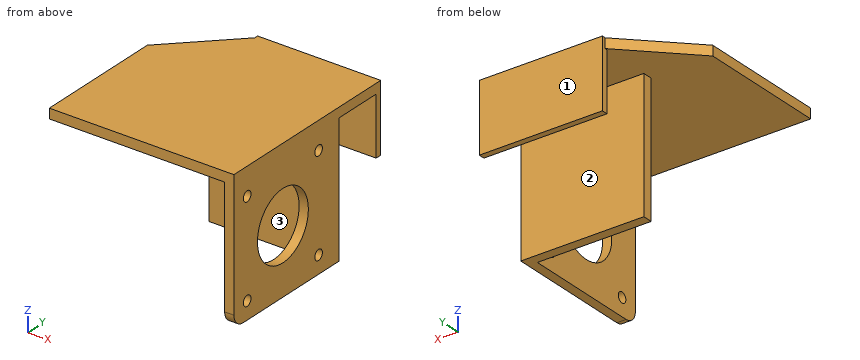
Solid Edge part; units mm, degrees
sketch "Sketch1" plane through (0, 0, 0) normal (1, 0, 0) x (0, 1, 0)
  circle A0 centre (-15.5, -15.5) radius 1.65
  circle A1 centre (0, 0) radius 11.05
  circle A2 centre (15.5, 15.5) radius 1.65
  line L0 (-21.25, 21.25) -> (21.25, 21.25)
  line L1 (21.25, 21.25) -> (21.25, -21.25)
  line L2 (21.25, -21.25) -> (-21.25, -21.25)
  line L3 (-21.25, -21.25) -> (-21.25, 21.25)
  circle A3 centre (-15.5, 15.5) radius 1.65
  circle A4 centre (15.5, -15.5) radius 1.65
extrude "Protrusion1" add sketch "Sketch1" against normal blind 3
sketch "Sketch2" plane through (0, 0, 0) normal (1, 0, 0) x (0, 1, 0)
  line L0 (24.45, -21.25) -> (21.25, -21.25)
  line L1 (21.25, 21.25) -> (21.25, -21.25)
  line L2 (21.25, 21.25) -> (21.25, 24.45)
  line L3 (-21.25, 24.45) -> (42.45, 24.45)
  line L4 (42.45, 24.45) -> (42.45, 2.25)
  line L5 (42.45, 2.25) -> (40.45, 2.25)
  line L6 (40.45, 2.25) -> (40.45, 21.25)
  line L7 (40.45, 21.25) -> (24.45, 21.25)
  line L8 (24.45, 21.25) -> (24.45, -21.25)
extrude "Fensterklammer" add sketch "Sketch2" against normal blind 40 material side at (0, 22.85, -21.2)
sketch "Sketch3" plane through (0, 0, 0) normal (1, 0, 0) x (0, 1, 0)
  line L0 (-21.25, 24.45) -> (42.45, 24.45)
  line L1 (21.25, 21.25) -> (21.25, 24.45)
  line L2 (-21.25, 21.25) -> (21.25, 21.25)
  line L3 (-21.25, 21.25) -> (-21.25, 24.45)
extrude "Elektonik_Halter" add sketch "Sketch3" against normal blind 60 material side at (0, 10.6, 24.4)
sketch "Sketch4" plane through (-31.5, 0, 21.25) normal (0, 0, -1) x (0, -1, 0)
  line L0 (-41.25, 8.5) -> (-21.25, 8.5)
  line L1 (-21.25, 8.5) -> (-21.25, 28.5)
  line L2 (-41.25, 8.5) -> (-21.25, 28.5)
extrude "Protrusion2" add sketch "Sketch4" against normal up to vertex (3.2 mm away)
fillet "R4" radius 4 1 edges at (-1.5, -21.25, -21.25)
Read the model definition and answer for the solid it produces. Units are mm, in the model's axes. Face numbers are marked on the shaded views. A direction names the side the tool comes from. Round coordinates to 2 decimals unless told otherwise and drop trailing zeros. Write each loop counter-clockwise with the first axis right and the second up, starting at its lowest first coordinate (ties: lowest second). Pieces come first, ordered by that corner, then holes.
1. The part is cut by section C-C, the plane z = -15.5. Determine the outline of the cut face in (x, y).
2. The part is cut by section D-D, the plane y = 0. Determine the outline of the cut face in (x, z).
3. Given pin 1 Ø3 at (y, z) = (-15.5, -15.5) entering from -X; pin 2 Ø6 at (y, z) = (-3, 18.5) entering from +X; pin 3 Ø1 at (x, y) = (-21.5, 41.5) entering from -Z; pin 4 Ø1.6 at (y, z) = (41.5, 17.5) entering from -X, each flat-ended and moving along its own axis, determine where each tip first touches the part or whether it passes through.
4. The part is cut by section A-A, the plane z = 19. Determine the outline of the cut face in (x, y), then the cut area to 4 significant figures.
5. Straight lines are drawn through the part: L1, parallel to Z at x = -1, y = 15.5; L2, parallel to Y at x = -2, z = -15; L3, parallel to Y at x = -39, z = 19.5. For each, find the intervals that lie inside material, in ascending order.
6. The part is cut by section B-B, the plane y = 15.5. Determine the outline of the cut face in (x, z), then the cut area to 3 significant figures.
7. Which of the six approach directions +Z, -Z, +X, -X, +Y, -Y give full straight-line access (tool end or side, diameter ignored) to the marked faces 1, 2 and 3?
Values:
1. outline: (-40, 21.25) - (-3, 21.25) - (-3, 17.15) - (0, 17.15) - (0, 24.45) - (-40, 24.45) - close; (-3, -21.25) - (0, -21.25) - (0, -17.15) - (-3, -17.15) - close; (-3, -13.85) - (0, -13.85) - (0, 13.85) - (-3, 13.85) - close
2. outline: (-60, 21.25) - (-3, 21.25) - (-3, 11.05) - (0, 11.05) - (0, 24.45) - (-60, 24.45) - close; (-3, -21.25) - (0, -21.25) - (0, -11.05) - (-3, -11.05) - close
3. pin 1: passes through
3. pin 2: stops at x = 0
3. pin 3: stops at z = 2.25
3. pin 4: stops at x = -40
4. outline: (-40, 21.25) - (-3, 21.25) - (-3, -21.25) - (0, -21.25) - (0, 24.45) - (-40, 24.45) - close; (-40, 40.45) - (0, 40.45) - (0, 42.45) - (-40, 42.45) - close
4. area: 335.5 mm2
5. L1: z = -21.25 to -17.15, -13.85 to 13.85, 17.15 to 24.45
5. L2: y = -21.25 to -17.07, -13.93 to 13.93, 17.07 to 24.45
5. L3: y = 21.25 to 24.45, 40.45 to 42.45
6. outline: (-60, 21.25) - (-3, 21.25) - (-3, 17.15) - (0, 17.15) - (0, 24.45) - (-60, 24.45) - close; (-3, -21.25) - (0, -21.25) - (0, -17.15) - (-3, -17.15) - close; (-3, -13.85) - (0, -13.85) - (0, 13.85) - (-3, 13.85) - close
6. area: 300 mm2
7. face 1: +Z, -Z, +X, -X, +Y
7. face 2: -Z, +X, -X
7. face 3: -Z, -X, -Y
